Here's the drawing with two shaded views (mm, measured from the low corner). I have some questions. Give positions to 0.01 mm unless a question says otherwise; leave off trailing zeros. Loops run counter-clockwise (first coordinate to the right, second up) from the corner with the lowest first, then second, coordinate; pieces in that order, holes last. Notation, with made-up numbers: (-17.75, 82.25) - (-7.75, 82.25) arc R5 ccw to (-7.75, 86.25) - close; hole circle Ø1 at (54.5, 26.5). An arc over 180 degrees is marked (long way). Write each question's results on one line, items separated by ' | '. Start each with the question number.
1) I want a section at B-B, the plane y = 5. Write out the boundary of the cut face in (x, z).
2) I want a section at C-C, the plane z = 2.25. Write out the boundary of the cut face in (x, y).
3) I'm going to push flat-ended pins straight in: pin 1 (3 mm diameter, centred on x = 3, y = 14.5, fed in from +Z) (1 decimal); pin 2 (2 mm diameter, centred on x = 7.5, y = 11.5, fed in from +Z) (1 decimal); pin 3 (4 mm diameter, centred on x = 3, z = 2.5, fed in from -Y). Where does each tip first touch, or does it pass through?
4) If I drill on probe 1 along Y at (x, z) = (4.25, 2.5); probe 2 along Z at (x, y) = (3, 14.5); probe 3 along X at (y, z) = (2.75, 2.5) (1 decimal), over which ranges is the centre line in solid material (lowest first)? Write a range as [from, to].
5) I want a section at A-A, the plane x = 4.5. Count the separate pieces of the cut face and the enclosed holes in it.
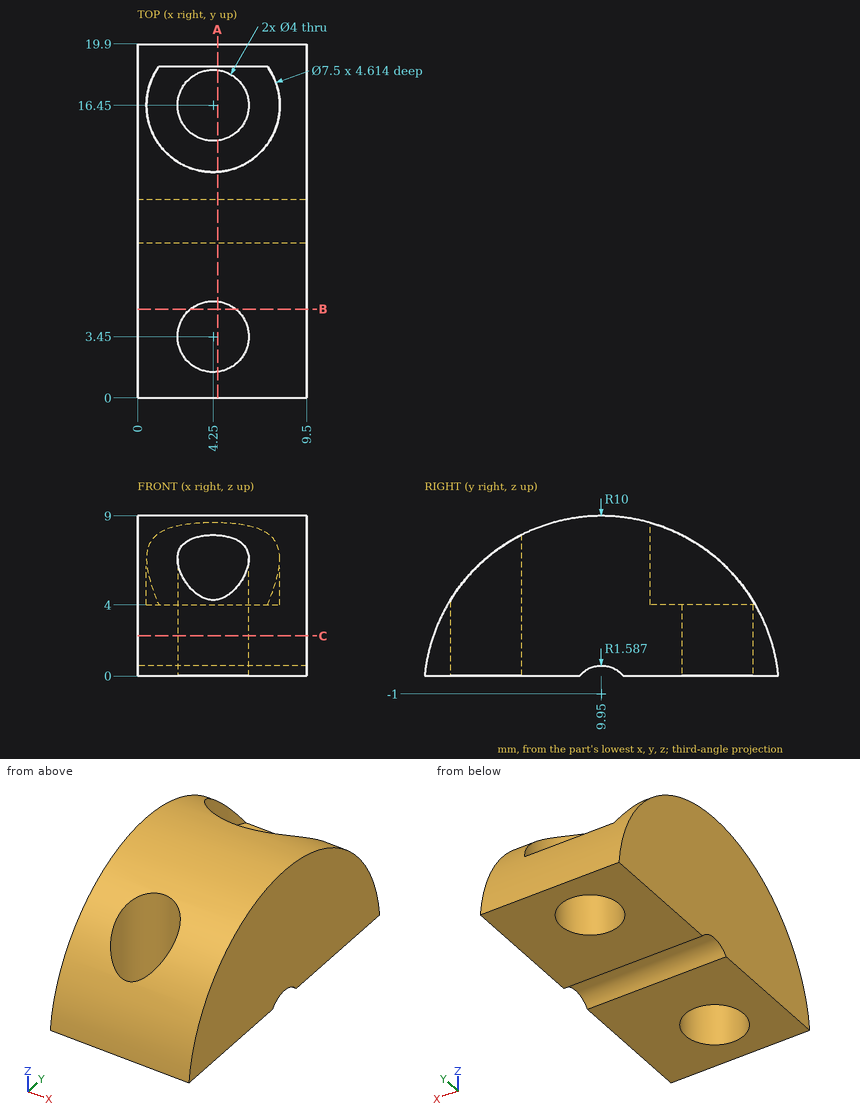
Answers:
1) outline: (0, 0) - (2.99, 0) - (2.99, 7.69) - (0, 7.69) - close; (5.51, 0) - (9.5, 0) - (9.5, 7.69) - (5.51, 7.69) - close
2) outline: (0, 0.49) - (9.5, 0.49) - (9.5, 19.41) - (0, 19.41) - close; hole circle Ø4 at (4.25, 3.45); hole circle Ø4 at (4.25, 16.45)
3) pin 1: stops at z = 8.5 | pin 2: stops at z = 9 | pin 3: stops at y = 0.06
4) probe 1: y = [0.58, 1.45], [5.45, 14.45], [18.45, 19.32] | probe 2: z = [0, 4] | probe 3: x = [0, 2.4], [6.1, 9.5]
5) separate pieces: 3 | enclosed holes: 0
